CAD build for the part. Positions are in the model's coordinates, mm. A direction names the side the tool comes from. Round coordinates to 2 decimals unless told otherwise and drop trailing zeros. Order: outer loops, then holes, each group sorted by start corner. A loop starts at its lowest first (then second) coordinate and runs counter-clockwise, first axis right, second up. Notation, with made-up numbers: (-39.75, -1.5) -> (-2.75, -1.5) arc R15 cw to (-2.75, 4.5) -> close; hole circle Ø3 at (75.5, 16.25). An arc over 180 degrees is marked (long way). Return JSON: item names as keys, results as strings. Group by question number.
Q1. Cut at B-B (x = 5.5). Write the cut outline in (y, z), then the cut area to 3 significant figures.
Q2. Cut at A-A (y = 43). Write the cut outline in (x, z), then the cut area to 3 significant figures.
Q3. Which spindle directions (+Z, -Z, +X, -X, +Y, -Y) get a long thin tool onto all of the face, cutting with end or side? Do faces 1 (the flat face through (-1, -8, 2)), 2 (the cylindrical face through (52.913, 60.424, 0.986)). Say none if no direction does.
Q4. Mould opens along Y. For faces 3 (the flat face through (-1, -8, 0)), 4 (the cylindrical face through (-53.283, 0.76, 0.986)), 5 (the cylindrical face through (-63.49, 52.45, 0.99)) say: +Y half, -Y half, draft (parallel to the pull), parting line (faces both ways), or undercut.
Q5. Probe line 1 along Y through (x, z) = (18, 1.8); line 2 along X through (y, z) = (37, 0.95); line 3 along Y through (x, z) = (0.5, 0.9). List the from-to ranges inside material, lowest first.
Q6. Cut at C-C (z = 1.7). Count the separate pieces of the cut face and the enclosed holes in it, then the cut area to 3 significant figures.
from build123d import *

# Parameters (mm, degrees)
SKETCH_1_R      = 1.5
SKETCH_1_W      = 8.2
SKETCH_1_H      = 2.2
SKETCH_1_W_2    = 2.2
SKETCH_1_H_2    = 8.2
EXTRUDE_1_DEPTH = 2


with BuildPart() as part:
    # 草图1 → 凸台-拉伸1 (new body)
    with BuildSketch(Plane.XY):
        Polygon((-68.061769393, -13.095981945), (-52.184883937, -13.095981945), (-18.934883937, -13.095981945), (18.565116063, -13.095981945), (67.695116063, -13.095981945), (67.695116063, 73.779018055), (1.315116063, 73.779018055), (1.315116063, 71.279018055), (2.815116063, 71.279018055), (2.815116063, 68.679018055), (1.315116063, 68.679018055), (1.315116063, 65.679018055), (-1.684883937, 65.679018055), (-1.684883937, 68.679018055), (-3.184883937, 68.679018055), (-3.184883937, 71.279018055), (-1.684883937, 71.279018055), (-1.684883937, 73.779018055), (-68.061769393, 73.779018055), align=None)
        with Locations((-33.184883937, -9.095981945)):
            Circle(SKETCH_1_R, mode=Mode.SUBTRACT)
        with Locations((-17.934883937, -9.095981946)):
            Rectangle(SKETCH_1_W, SKETCH_1_H, mode=Mode.SUBTRACT)
        with Locations((-64.184883937, 22.341518055)):
            Rectangle(SKETCH_1_W_2, SKETCH_1_H_2, mode=Mode.SUBTRACT)
        with Locations((17.565116063, -9.095981946)):
            Rectangle(SKETCH_1_W, SKETCH_1_H, mode=Mode.SUBTRACT)
        with Locations((32.815116063, -9.095981945)):
            Circle(SKETCH_1_R, mode=Mode.SUBTRACT)
        with Locations((63.815116063, 22.341518055)):
            Rectangle(SKETCH_1_W_2, SKETCH_1_H_2, mode=Mode.SUBTRACT)
        with BuildLine():
            ThreePointArc((50.815116063, 61.279018055), (52.936436406, 60.400338398), (53.815116063, 58.279018055))
            Line((53.815116063, 58.279018055), (53.815116063, 2.904018055))
            ThreePointArc((53.815116063, 2.904018055), (52.936436406, 0.782697711), (50.815116063, -0.095981945))
            Line((50.815116063, -0.095981945), (-51.184883937, -0.095981945))
            ThreePointArc((-51.184883937, -0.095981945), (-53.306204281, 0.782697711), (-54.184883937, 2.904018055))
            Line((-54.184883937, 2.904018055), (-54.184883937, 58.279018055))
            ThreePointArc((-54.184883937, 58.279018055), (-53.306204281, 60.400338398), (-51.184883937, 61.279018055))
            Line((-51.184883937, 61.279018055), (50.815116063, 61.279018055))
        make_face(mode=Mode.SUBTRACT)
        with Locations((-64.184883937, 53.779018055)):
            Circle(SKETCH_1_R, mode=Mode.SUBTRACT)
        with Locations((63.815116063, 53.779018055)):
            Circle(SKETCH_1_R, mode=Mode.SUBTRACT)
    extrude(amount=EXTRUDE_1_DEPTH)


solid = part.part
Solution:
{
 "1": {"outline": "(-13.1, 0) -> (-0.1, 0) -> (-0.1, 2) -> (-13.1, 2) -> close; (61.28, 0) -> (73.78, 0) -> (73.78, 2) -> (61.28, 2) -> close", "area": "51.0 mm²"},
 "2": {"outline": "(-68.06, 0) -> (-54.18, 0) -> (-54.18, 2) -> (-68.06, 2) -> close; (53.82, 0) -> (67.7, 0) -> (67.7, 2) -> (53.82, 2) -> close", "area": "55.5 mm²"},
 "3": {"face 1": "+Z, +X, -X, +Y, -Y", "face 2": "+Z, -Z"},
 "4": {"face 3": "draft", "face 4": "undercut", "face 5": "undercut"},
 "5": {"line 1": "y = -13.1 to -10.2, -8 to -0.1, 61.28 to 73.78", "line 2": "x = -68.06 to -54.18, 53.82 to 67.7", "line 3": "y = -13.1 to -0.1, 61.28 to 65.68"},
 "6": {"separate pieces": "1", "enclosed holes": "9", "area": "5,040 mm²"}
}
